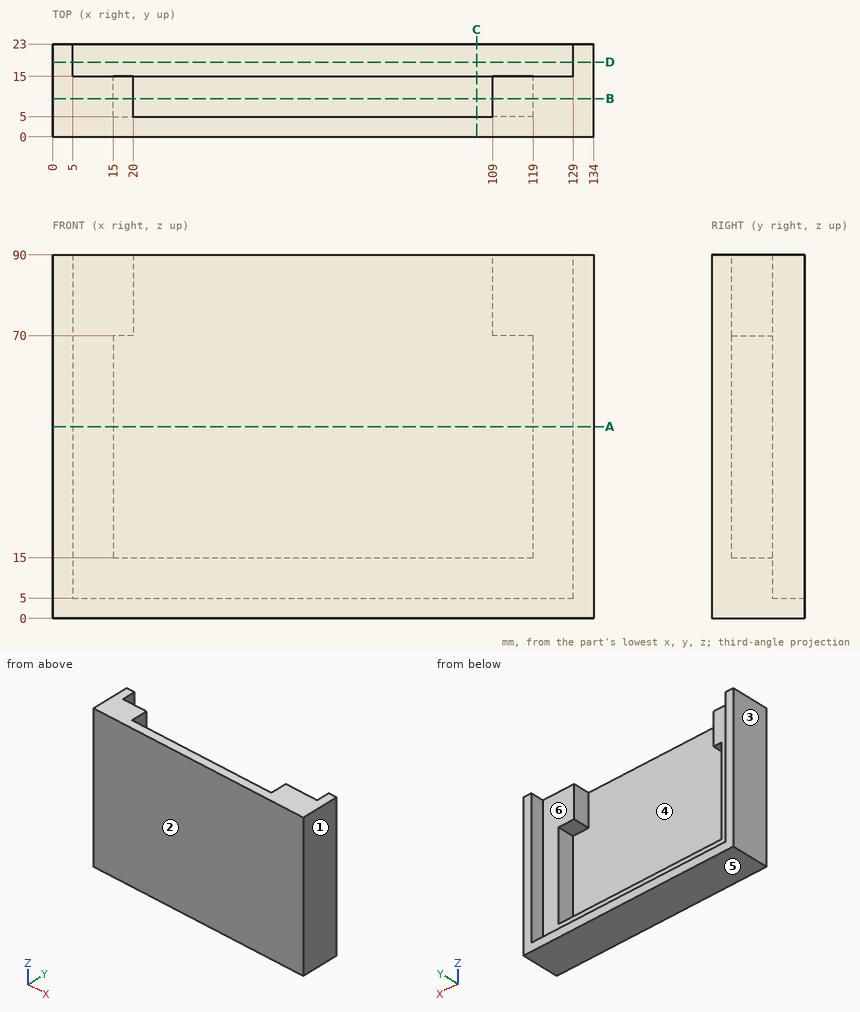
For this review, use the dimensioned drawing (mm, ordinates from the lowest corner) and the shaded views. A direction names the side the tool comes from. Coordinates: 2 decimals unless noted, no trailing zeros. Order: outer loops, then holes, each group sorted by start corner. A loop starts at its lowest first (then second) coordinate and runs counter-clockwise, first axis right, second up. Notation, with made-up numbers: (-28.75, 7) - (27.25, 7) arc R12 cw to (27.25, 28) - close; hole circle Ø2 at (-18.75, 73.25). An arc over 180 degrees is marked (long way). Answer in a Markdown table with one row per item.
(1) Clearance check with flat-ended pins moving along their axes: pin 1 (3 mm diameter, centred on x = 91, y = 10.5, fed in from +Z); pin 2 (6.5 mm diameter, centred on x = 87.5, y = 20.5, fed in from +Z); pin 3 (6 mm diameter, centred on x = 43, z = 49.5, fed in from +Y). State where each tip first meets the part, or that it passes through.
Checked values:
| item | result |
|---|---|
| pin 1 | z = 15 |
| pin 2 | z = 5 |
| pin 3 | y = 5 |
(2) For the marked faces 5 and 6, list the 3-axis set-ups (+Z, -Z, +X, -X, +Y, -Y) from which the entire face can be reached by the end or side of a thin tool; tool diameter is ignored.
Checked values:
| item | result |
|---|---|
| face 5 | -Z, +X, -X, +Y, -Y |
| face 6 | +Z, +Y |
(3) Consider section D-D on y = 18.5. State the section outline as (x, z) points.
Checked values:
| item | result |
|---|---|
| outline | (0, 0) - (134, 0) - (134, 90) - (129, 90) - (129, 5) - (5, 5) - (5, 90) - (0, 90) - close |
(4) Consider section B-B on y = 9.5. State the section outline as (x, z) points.
Checked values:
| item | result |
|---|---|
| outline | (0, 0) - (134, 0) - (134, 90) - (109, 90) - (109, 70) - (119, 70) - (119, 15) - (15, 15) - (15, 70) - (20, 70) - (20, 90) - (0, 90) - close |
(5) Consider section C-C on x = 105. State the section outline as (y, z) points.
Checked values:
| item | result |
|---|---|
| outline | (0, 0) - (23, 0) - (23, 5) - (15, 5) - (15, 15) - (5, 15) - (5, 90) - (0, 90) - close |
(6) Wall thickness on line 1 along X through (y, z) = (15.5, 61); line 2 along Z through (x, y) = (117, 14.5); line 3 along X through (y, z) = (9.75, 56.5): over which ranges is each line inside the solid? List them lowest first. Write a range as from..to.
Checked values:
| item | result |
|---|---|
| line 1 | 0..5, 129..134 |
| line 2 | 0..15, 70..90 |
| line 3 | 0..15, 119..134 |
(7) Consider section A-A on z = 47.5. State the section outline as (x, y) points.
Checked values:
| item | result |
|---|---|
| outline | (0, 0) - (134, 0) - (134, 23) - (129, 23) - (129, 15) - (119, 15) - (119, 5) - (15, 5) - (15, 15) - (5, 15) - (5, 23) - (0, 23) - close |
(8) The part is to be moulded in two halves that separate along X. For the marked faces 1, 2, 3 and 4, say which applies: released by +X, released by -X, zero draft, split by the parting line, or undercut.
Checked values:
| item | result |
|---|---|
| face 1 | released by +X |
| face 2 | zero draft |
| face 3 | released by -X |
| face 4 | undercut |
